Can you work these out from the model? Positions are in its coordinate system, mm. Face numbers are marked on the shaded views. A direction names the side the tool comes from. Give positions to 0.01 mm unless a question says otherwise; leave off trailing zeros. Order: outer loops, then holes, each group sorted by start corner. A loop starts at its lowest first (then second) coordinate and runs counter-clockwise, first axis right, second up. Notation, with made-up numbers: M -22,-39 L 36,-39 A18 cw 36,-17 Z; hole C 57.5,-26.75 d11. An arc over 180 degrees is marked long. Use a Markdown table: item, result. Add a question column.
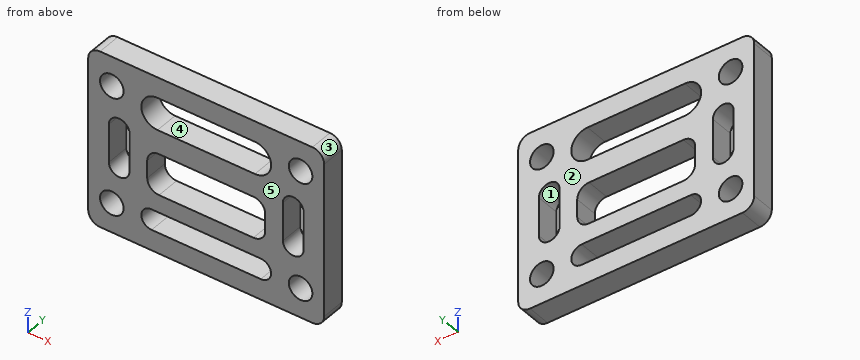
from build123d import *

# Parameters (mm, degrees)
SKETCH_1_W          = 40
SKETCH_1_H          = 30
SKETCH_1_R          = 2
SKETCH_1_W_2        = 20
SKETCH_1_H_2        = 7
EXTRUDE_1_DEPTH     = 4
CUT_EXTRUDE_1_DEPTH = 26.317977802
FILLET_1_R          = 2


with BuildPart() as part:
    # 草图1 → 凸台-拉伸1 (new body)
    with BuildSketch(Plane(origin=(0, 0, 0), x_dir=(1, 0, 0), z_dir=(0, 1, 0))):
        Rectangle(SKETCH_1_W, SKETCH_1_H)
        with Locations(Location((-16, 10, 0), (0, 0, 270))):
            Circle(SKETCH_1_R, mode=Mode.SUBTRACT)
        with Locations(Location((-16, -10, 0), (0, 0, 270))):
            Circle(SKETCH_1_R, mode=Mode.SUBTRACT)
        with Locations(Location((16, 10, 0), (0, 0, 270))):
            Circle(SKETCH_1_R, mode=Mode.SUBTRACT)
        with Locations(Location((16, -10, 0), (0, 0, 270))):
            Circle(SKETCH_1_R, mode=Mode.SUBTRACT)
        with Locations((0, 1.5)):
            Rectangle(SKETCH_1_W_2, SKETCH_1_H_2, mode=Mode.SUBTRACT)
    extrude(amount=EXTRUDE_1_DEPTH)

    # 草图2 → 切除-拉伸1 (cut, through all)
    with BuildSketch(Plane(origin=(0, 4, 0), x_dir=(1, 0, 0), z_dir=(0, 1, 0))):
        with BuildLine():
            Line((-9.25, 11.5), (9.25, 11.5))
            ThreePointArc((9.25, 11.5), (11, 9.75), (9.25, 8))
            Line((9.25, 8), (-9.25, 8))
            ThreePointArc((-9.25, 8), (-11, 9.75), (-9.25, 11.5))
        make_face()
        with BuildLine():
            Line((-13, 3.25), (-13, -3.25))
            ThreePointArc((-13, -3.25), (-14.75, -5), (-16.5, -3.25))
            Line((-16.5, -3.25), (-16.5, 3.25))
            ThreePointArc((-16.5, 3.25), (-14.75, 5), (-13, 3.25))
        make_face()
        with BuildLine():
            Line((13, 3.25), (13, -3.25))
            ThreePointArc((13, -3.25), (14.75, -5), (16.5, -3.25))
            Line((16.5, -3.25), (16.5, 3.25))
            ThreePointArc((16.5, 3.25), (14.75, 5), (13, 3.25))
        make_face()
        with BuildLine():
            Line((-8.25, -11.5), (8.25, -11.5))
            ThreePointArc((8.25, -11.5), (11, -8.75), (8.25, -6))
            Line((8.25, -6), (-8.25, -6))
            ThreePointArc((-8.25, -6), (-11, -8.75), (-8.25, -11.5))
        make_face()
    extrude(amount=-CUT_EXTRUDE_1_DEPTH, mode=Mode.SUBTRACT)

    # 圆角1
    fillet_1_edges = [part.edges().sort_by_distance(p)[0] for p in [
        (-10, 2, -5),
        (-10, 2, 2),
        (10, 2, 2),
        (10, 2, -5),
        (-20, 2, -15),
        (20, 2, -15),
        (20, 2, 15),
        (-20, 2, 15),
    ]]
    fillet(fillet_1_edges, radius=FILLET_1_R)


solid = part.part
1. If we section it at D-D, the plane y = 2: State how many separate pieces and enclosed holes the cut face has, then the cut area to 3 significant figures.
2. If we section it at C-C, the plane x = 10.5: List the corners of the cut face in (y, z) for me, then the cut area to 3 significant figures.
3. I need wall thicknesses on L1, parallel to Z at x = -4, y = 1.75; L2, parallel to X at y = 2.95, z = -2; L3, parallel to X at y = 2.35, z = 10. Which ranges of each line are inside material? Lowest first, please. Write a range as [from, to].
4. We'd pull the mould along Z, two halves only. Please class the marked faces 1, 2 and 3: +Z half, -Z half, draft (parallel to the pull), parting line (faces both ways), or undercut.
5. On a 3-axis mill with a long thin cutter (end or side, diameter ignored), from which of +Z, -Z, +X, -X, +Y, -Y can I reach the whole of each face in a straight line? I mean the marked faces 4 and 5. Say none if no direction works.
6. Will this pin go through, and if not, where does the flat tip stop? pin 1 (2.5 mm diameter, centred on x = -16, z = 10, fed in from +Y).
7. If we section it at B-B, the plane z = -8.5: List the corners of the cut face in (x, y) for me.
8. If we section it at A-A, the plane x = 4.5: List the corners of the cut face in (y, z) for me, then the cut area to 3 significant figures.
Geometry results:
| question | item | result |
|---|---|---|
| 1 | separate pieces | 1 |
| 1 | enclosed holes | 9 |
| 1 | area | 756 mm^2 |
| 2 | outline | M 0,-15 L 4,-15 L 4,-10.97 L 0,-10.97 Z; M 0,-8.53 L 4,-8.53 L 4,7.17 L 0,7.17 Z; M 0,10.33 L 4,10.33 L 4,15 L 0,15 Z |
| 2 | area | 97.6 mm^2 |
| 3 | L1 | z = [-15, -11.5], [-8, -5], [2, 6], [11.5, 15] |
| 3 | L2 | x = [-20, -16.5], [-13, -10], [10, 13], [16.5, 20] |
| 3 | L3 | x = [-20, -18], [-14, -10.7], [10.7, 14], [18, 20] |
| 4 | face 1 | undercut |
| 4 | face 2 | draft |
| 4 | face 3 | +Z half |
| 5 | face 4 | +Y, -Y |
| 5 | face 5 | +Z, -Z, +X, -X, -Y |
| 6 | pin 1 | passes through |
| 7 | outline | M -20,0 L -17.32,0 L -17.32,4 L -20,4 Z; M -14.68,0 L -10.47,0 L -10.47,4 L -14.68,4 Z; M 10.47,0 L 14.68,0 L 14.68,4 L 10.47,4 Z; M 17.32,0 L 20,0 L 20,4 L 17.32,4 Z |
| 8 | outline | M 0,-15 L 4,-15 L 4,-11.5 L 0,-11.5 Z; M 0,-8 L 4,-8 L 4,-5 L 0,-5 Z; M 0,2 L 4,2 L 4,6 L 0,6 Z; M 0,11.5 L 4,11.5 L 4,15 L 0,15 Z |
| 8 | area | 56.0 mm^2 |
